```python
from build123d import *

# Parameters (mm, degrees)
BOSS_EXTRUDE1_DEPTH = 88.9
FILLET1_R           = 1.9812
FILLET2_R           = 3.9624
FILLET3_R           = 6.35
SKETCH2_R           = 3.3782
CUT_EXTRUDE1_DEPTH  = 88.9


with BuildPart() as part:
    # Sketch1 → Boss-Extrude1 (new body)
    with BuildSketch(Plane(origin=(0, 0, 0), x_dir=(0, 0, -1), z_dir=(1, 0, 0))):
        Polygon((0, 44.45), (0, 0), (44.45, 0), (44.45, 1.9812), (1.9812, 1.9812), (1.9812, 44.45), align=None)
    extrude(amount=BOSS_EXTRUDE1_DEPTH)

    # Fillet1
    fillet1_edges = [part.edges().sort_by_distance(p)[0] for p in [
        (44.45, 1.9812, -1.9812),
    ]]
    fillet(fillet1_edges, radius=FILLET1_R)

    # Fillet2
    fillet2_edges = [part.edges().sort_by_distance(p)[0] for p in [
        (44.45, 0, 0),
    ]]
    fillet(fillet2_edges, radius=FILLET2_R)

    # Fillet3
    fillet3_edges = [part.edges().sort_by_distance(p)[0] for p in [
        (88.9, 0.9906, -44.45),
        (88.9, 44.45, -0.9906),
        (0, 0.9906, -44.45),
        (0, 44.45, -0.9906),
    ]]
    fillet(fillet3_edges, radius=FILLET3_R)

    # Sketch2 → Cut-Extrude1 (cut)
    with BuildSketch(Plane.XY):
        with Locations((12.7, 22.225)):
            Circle(SKETCH2_R)
        with Locations((76.2, 22.225)):
            Circle(SKETCH2_R)
    extrude(amount=-CUT_EXTRUDE1_DEPTH, mode=Mode.SUBTRACT)


solid = part.part
```
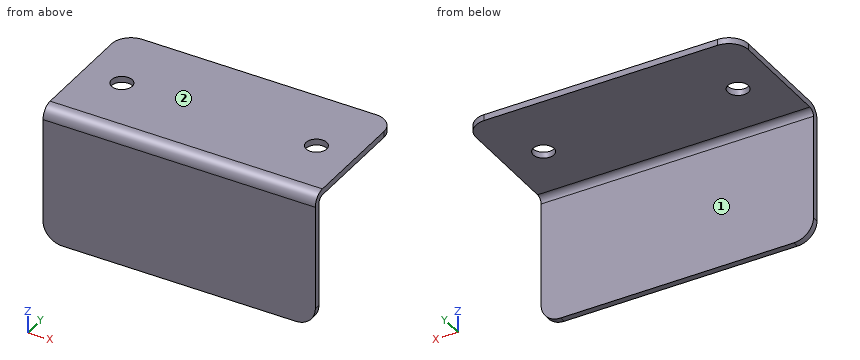
For this review, take the finished solid that the model builds, in its own axes (mm). Face numbers are marked on the shaded views. A direction names the side the tool comes from. Coordinates: 2 decimals unless noted, no trailing zeros. Loops run counter-clockwise (first coordinate to the right, second up) from the corner with the lowest first, then second, coordinate; pieces in that order, holes last.
1. For line 1 (Z direction, x = 56.5, y = 42); line 2 (Y direction, x = 56.5, z = -20); line 3 (Y direction, x = 76.2, z = -1.5), list the stretches that pass through material, from the lowest coordinate up.
2. Add section B-B, the plane y = 24. Give the boundary of the cut face in (x, z), then the cut area to 3 significant figures.
3. Add section D-D, the plane y = 5. Give the boundary of the cut face in (x, z), then the cut area to 3 significant figures.
4. Add section A-A, the plane x = 76.2. Give the boundary of the cut face in (y, z).
5. For the marked faces 1 and 2, list the 3-axis set-ups (+Z, -Z, +X, -X, +Y, -Y) from which the entire face can be reached by the end or side of a thin tool; tool diameter is ignored.
6. Insertion check: P1, Ø12, axis at x = 48.5, z = -18, coming from the +Y side; P2, Ø6, axis at x = 12.7, y = 22.225, coming from the +Z side; P3, Ø8, axis at x = 76.2, y = 22.225, coming from the -Z side. Each pin has a flat end and moves straight along its axis. Give the tip position at first contact, or say it passes through.
7. Add section C-C, the plane x = 44. Give the boundary of the cut face in (y, z).
Result:
1. line 1: z = -1.98 to 0
1. line 2: y = 0 to 1.98
1. line 3: y = 0.86 to 18.85, 25.6 to 44.45
2. outline: (0, -1.98) - (9.83, -1.98) - (9.83, 0) - (0, 0) - close; (15.57, -1.98) - (73.33, -1.98) - (73.33, 0) - (15.57, 0) - close; (79.07, -1.98) - (88.9, -1.98) - (88.9, 0) - (79.07, 0) - close
2. area: 153 mm2
3. outline: (0, -1.98) - (88.9, -1.98) - (88.9, 0) - (0, 0) - close
3. area: 176 mm2
4. outline: (0, -44.45) - (1.98, -44.45) - (1.98, -3.96) arc R1.98 cw to (3.96, -1.98) - (18.85, -1.98) - (18.85, 0) - (3.96, 0) arc R3.96 ccw to (0, -3.96) - close; (25.6, -1.98) - (44.45, -1.98) - (44.45, 0) - (25.6, 0) - close
5. face 1: -Z, +X, -X, +Y
5. face 2: +Z, +X, -X, +Y, -Y
6. P1: stops at y = 1.98
6. P2: passes through
6. P3: stops at z = -1.98
7. outline: (0, -44.45) - (1.98, -44.45) - (1.98, -3.96) arc R1.98 cw to (3.96, -1.98) - (44.45, -1.98) - (44.45, 0) - (3.96, 0) arc R3.96 ccw to (0, -3.96) - close
